Input: dimensioned drawing with shaded views. Units: mm. Origin: part minimum x, y, z. Give positions to 0.01 mm unless a question says otherwise; leave off trailing zeros. Loops run counter-clockwise (first coordinate to the right, second up) from the corner with the lowest first, then second, coordinate; pieces in that order, holes last. Notation, with made-up numbers: (21, 77) -> (70, 77) arc R13 ccw to (70, 87) -> close; hole circle Ø3 at (-30.5, 9.25). An arc over 180 degrees is marked (long way). One line per question, with ' | ' between items. Start each with the question number.
Item 1: Material intervals for line 1 along Y through (x, z) = (64.5, 0.85); line 2 along X through (y, z) = (45, 0.7); line 3 along Y through (x, z) = (80, 1.4), sorted ascending. Write a range as [from, to].
Item 2: Section B-B on y = 46. Return loops of the section in (x, z), then the cut area to 3 significant figures.
Item 3: Pin query (flat end, axial travel): P1, Ø1.5, axis at x = 91.5, z = 1, coming from the +Y side; P2, Ø0.9, axis at y = 27.5, z = 1, coming from the -X side; P3, Ø0.9, axis at y = 19.5, z = 2, coming from the +X side. Return the tip coordinate at first contact, or that it passes through.
Item 4: Section D-D on x = 61. Return loops of the section in (y, z), then the cut area to 3 significant figures.
Item 5: Section A-A on x = 29. Return loops of the section in (y, z), then the cut area to 3 significant figures.
Item 6: Section C-C on z = 1.1. Return loops of the section in (x, y).
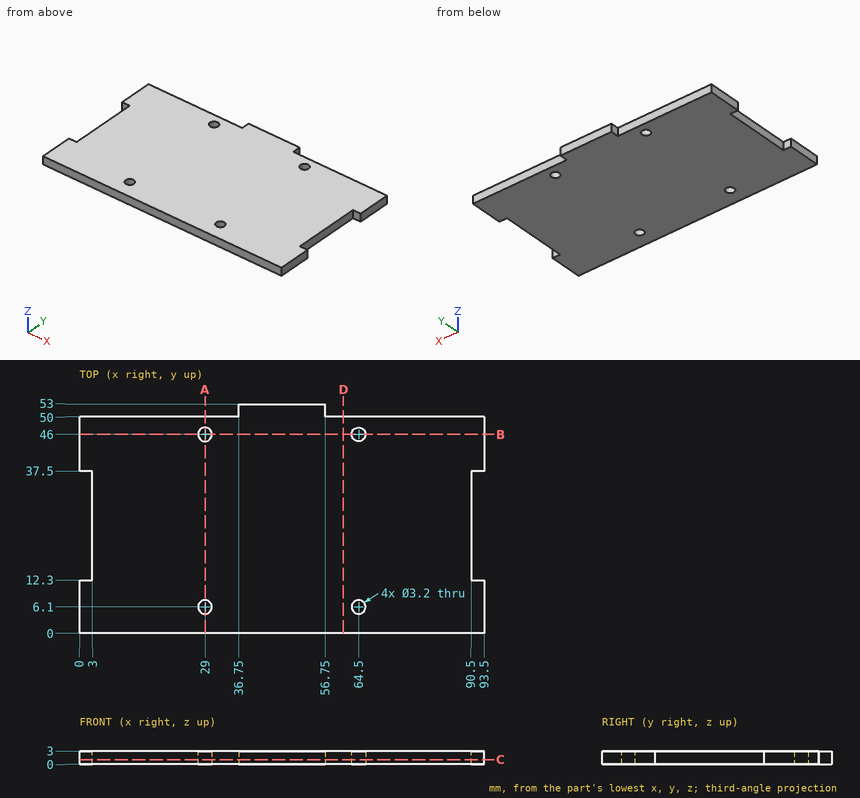
Result sheet:
1) line 1: y = [0, 4.5], [7.7, 44.4], [47.6, 50] | line 2: x = [0, 27.75], [30.25, 63.25], [65.75, 93.5] | line 3: y = [0, 50]
2) outline: (0, 0) -> (27.4, 0) -> (27.4, 3) -> (0, 3) -> close; (30.6, 0) -> (62.9, 0) -> (62.9, 3) -> (30.6, 3) -> close; (66.1, 0) -> (93.5, 0) -> (93.5, 3) -> (66.1, 3) -> close | area: 261 mm²
3) P1: stops at y = 50 | P2: stops at x = 3 | P3: stops at x = 90.5
4) outline: (0, 0) -> (50, 0) -> (50, 3) -> (0, 3) -> close | area: 150 mm²
5) outline: (0, 0) -> (4.5, 0) -> (4.5, 3) -> (0, 3) -> close; (7.7, 0) -> (44.4, 0) -> (44.4, 3) -> (7.7, 3) -> close; (47.6, 0) -> (50, 0) -> (50, 3) -> (47.6, 3) -> close | area: 131 mm²
6) outline: (0, 0) -> (93.5, 0) -> (93.5, 12.3) -> (90.5, 12.3) -> (90.5, 37.5) -> (93.5, 37.5) -> (93.5, 50) -> (56.75, 50) -> (56.75, 53) -> (36.75, 53) -> (36.75, 50) -> (0, 50) -> (0, 37.5) -> (3, 37.5) -> (3, 12.3) -> (0, 12.3) -> close; hole circle Ø3.2 at (29, 6.1); hole circle Ø3.2 at (29, 46); hole circle Ø3.2 at (64.5, 6.1); hole circle Ø3.2 at (64.5, 46)
